Can you work these out from the model? Positions are in its coordinate system, mm. Face numbers are marked on the shaded views. Round coordinates to 2 decimals unless told otherwise and drop trailing zeros. Order: outer loops, then holes, each group sorted by start corner. A loop starts at its lowest first (then second) coordinate and runs counter-clockwise, first axis right, second up. Notation, with made-up numbers: M 35.25,24.25 L 63.25,24.25 A17 cw 63.25,31.25 Z; hole C 5,-4 d4. An arc over 180 degrees is marked long. Answer as a JSON object with one key per item and string values. Group by question number.
```python
from build123d import *

# Parameters (mm, degrees)
F0_W     = 86.277299
F0_H     = 69.66754
F1_DEPTH = 25.4
F2_R     = 5.08
F3_R     = 5
F4_R     = 5
F5_R     = 5
F7_D     = 5


with BuildPart() as f1:
    # F0 (on Right) → F1 (new body)
    with BuildSketch(Plane.YZ):
        with Locations((10.387514, -5.193766)):
            Rectangle(F0_W, F0_H)
    extrude(amount=F1_DEPTH)

    # F2
    f2_edges = [f1.edges().sort_by_distance(p)[0] for p in [
        (25.4, 10.387514, -40.027536),
    ]]
    fillet(f2_edges, radius=F2_R)

    # F3
    f3_edges = [f1.edges().sort_by_distance(p)[0] for p in [
        (25.4, 53.526163, -2.653766),
    ]]
    fillet(f3_edges, radius=F3_R)

    # F4
    f4_edges = [f1.edges().sort_by_distance(p)[0] for p in [
        (25.4, 7.887514, 29.640004),
    ]]
    fillet(f4_edges, radius=F4_R)

    # F5
    f5_edges = [f1.edges().sort_by_distance(p)[0] for p in [
        (25.4, -32.751136, -5.153766),
    ]]
    fillet(f5_edges, radius=F5_R)

    # F7 (through all)
    with Locations(Plane.YZ.offset(25.4)):
        with Locations((-14.6505, 0)):
            Hole(F7_D / 2)


solid = f1.part
```
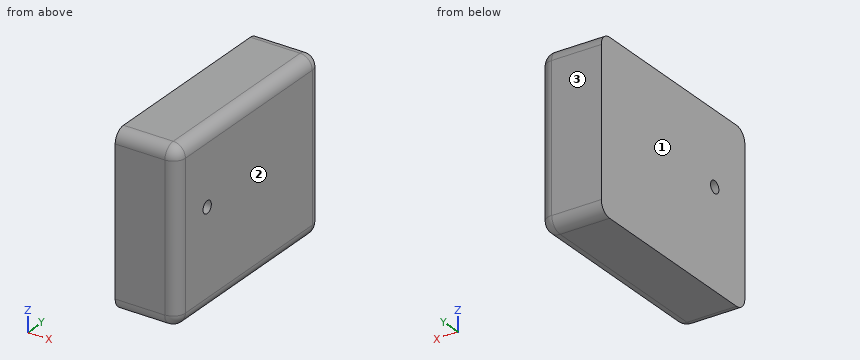
1) I need wall thicknesses on line 1 along X through (y, z) = (47, 26); line 2 along X through (y, z) = (4.5, 26.5); line 3 along Z through (x, y) = (23.25, 29). Which ranges of each line are inside material? Lowest first, please.
2) We'd pull the mould along X, two halves only. Please class the marked faces 1, 2 and 3: +X half, -X half, draft (parallel to the pull), parting line (faces both ways), or undercut.
3) If we section it at A-A on z = 0: Write out the boundary of the cut face in (x, y).
Findings:
{
 "1": {"line 1": "x = 0 to 25.21", "line 2": "x = 0 to 25.04", "line 3": "z = -39.1 to 28.75"},
 "2": {"face 1": "-X half", "face 2": "+X half", "face 3": "draft"},
 "3": {"outline": "M 0,-32.75 L 20.4,-32.75 A5 ccw 25.4,-27.75 L 25.4,-17.15 L 0,-17.15 Z; M 0,-12.15 L 25.4,-12.15 L 25.4,48.53 A5 ccw 20.4,53.53 L 0,53.53 Z"}
}
